Geometry check sheet. Reference: the model listing, model coordinates, mm. Face numbers are marked on the shaded views. A direction names the side the tool comes from. Round coordinates to 2 decimals unless told otherwise and drop trailing zeros. Order: outer loops, then holes, each group sorted by start corner. A loop starts at its lowest first (then second) coordinate and runs counter-clockwise, first axis right, second up.
(1) Sectioned sample at C-C (y = 5.25). Record the boundary of the cut face in (x, z), plus the area to 3 significant figures.
(2) Release check for a two-part mould opening along X. For the marked faces 3, 4 and 5 record: +X half, -X half, draft (parallel to the pull), parting line (faces both ways), or undercut.
(3) Go/stop test with flat-tipped pins: pin 1 (4 mm diameter, centred on x = -5, y = 10, fed in from -Z); pin 2 (1.5 mm diameter, centred on y = 16, z = 7, fed in from -X); pin 3 (12 mm diameter, centred on y = 7, z = -10, fed in from -X). Record where each tip stops, or that it passes through.
(4) Material ranges on line 1 along X through (y, z) = (1.1, 0); line 2 along Z through (x, y) = (0, 15.65), recorded low to high.
(5) Set-up check for the marked faces 1 and 2: record each of +Z, -Z, +X, -X, +Y, -Y from which the full face is reachable in a straight line by a thin tool's end or side.
(6) Sectioned sample at D-D (y = 18.75). Record the boundary of the cut face in (x, z), plus the area to 3 significant figures.
from build123d import *

# Parameters (mm, degrees)
CHAMFER_1_SIZE = 0.5


with BuildPart() as part:
    # Эскиз1 → Повернуть1 (revolve)
    with BuildSketch(Plane.XY):
        Polygon((17, 0), (17, 2), (21, 2), (21, 15), (22.25, 15), (22.25, 17.15), (21, 17.15), (21, 20), (25, 20), (25, 6.5), (27.5, 6.5), (27.5, 4), (25, 4), (25, 0), align=None)
    revolve(axis=Axis((0, 0, 0), (0, 1, 0)))

    # Фаска1
    chamfer_1_edges = [part.edges().sort_by_distance(p)[0] for p in [
        (-25, 20, 0),
        (-21, 20, 0),
    ]]
    chamfer(chamfer_1_edges, length=CHAMFER_1_SIZE)


solid = part.part
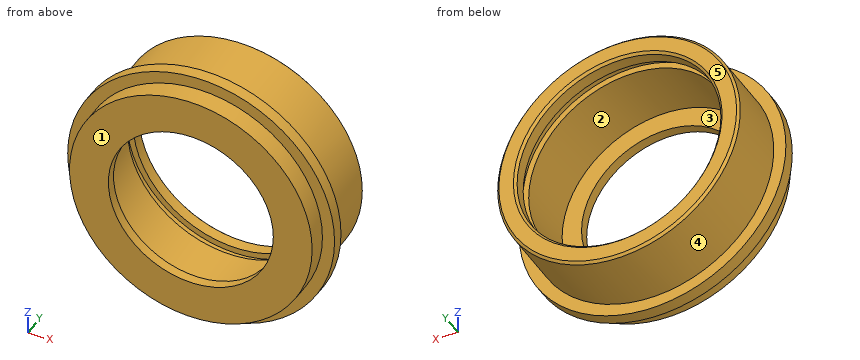
Answer below:
1. outline: circle Ø55 at (0, 0); hole circle Ø42 at (0, 0)
1. area: 990 mm2
2. face 3: undercut
2. face 4: parting line
2. face 5: draft
3. pin 1: stops at z = -24.82
3. pin 2: stops at x = -24.21
3. pin 3: stops at x = -27.2
4. line 1: x = -25 to -17, 17 to 25
4. line 2: z = -25 to -22.25, 22.25 to 25
5. face 1: +Z, -Z, +X, -X, -Y
5. face 2: +Y
6. outline: circle Ø50 at (0, 0); hole circle Ø42 at (0, 0)
6. area: 578 mm2
